Geometry check sheet. Reference: drawing and pictorial views, mm from the part's lowest x, y, z. Give positions to 0.01 mm unless a question says otherwise; leave off trailing zeros. Loops run counter-clockwise (first coordinate to the right, second up) from the corner with the lowest first, then second, coordinate; pieces in that order, holes last. Notation, with made-up numbers: (34, -13) - (71, -13) arc R25 ccw to (71, 17) - close; hole circle Ø8 at (16, -28). An arc over 180 degrees is marked (long way). One line per question, with ' | ' between items. Start each with the question number.
1. Depth check by flat-ended pin: pin 1 Ø2.5 at (x, z) = (50.9, 32) entering from -Y. Enter the tip coordinate at first touch or a pass-through.
2. Section check D-D, the plane y = 0.65. Enter the section's corners in (x, z).
3. Section check B-B, the plane z = 3. Enter the section's corners in (x, y), then the cut area to 3 significant figures.
4. Section check A-A, the plane x = 50.9. Enter the section's corners in (y, z), then the cut area to 3 significant figures.
5. Thickness scan on line 1 along X through (y, z) = (0.7, 32); line 2 along Z through (x, y) = (3.1, 0.6); line 3 along Z through (x, y) = (46.5, 0.4). Record the ranges inside material, lowest first. Write a range as from..to.
6. Section check C-C, the plane x = 3.1. Enter the section's corners in (y, z).
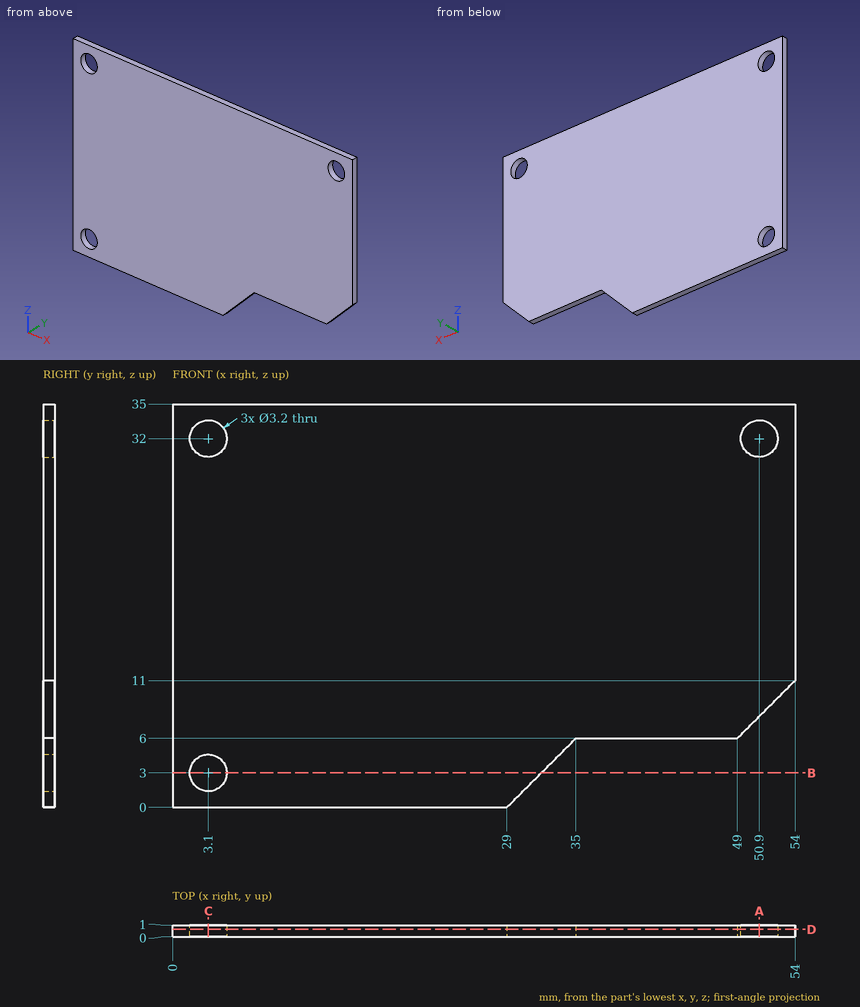
Results list:
1) pin 1: through
2) outline: (0, 0) - (29, 0) - (35, 6) - (49, 6) - (54, 11) - (54, 35) - (0, 35) - close; hole circle Ø3.2 at (3.1, 3); hole circle Ø3.2 at (3.1, 32); hole circle Ø3.2 at (50.9, 32)
3) outline: (0, 0) - (1.5, 0) - (1.5, 1) - (0, 1) - close; (4.7, 0) - (32, 0) - (32, 1) - (4.7, 1) - close | area: 28.8 mm²
4) outline: (0, 7.9) - (1, 7.9) - (1, 30.4) - (0, 30.4) - close; (0, 33.6) - (1, 33.6) - (1, 35) - (0, 35) - close | area: 23.9 mm²
5) line 1: 0..1.5, 4.7..49.3, 52.5..54 | line 2: 0..1.4, 4.6..30.4, 33.6..35 | line 3: 6..35
6) outline: (0, 0) - (1, 0) - (1, 1.4) - (0, 1.4) - close; (0, 4.6) - (1, 4.6) - (1, 30.4) - (0, 30.4) - close; (0, 33.6) - (1, 33.6) - (1, 35) - (0, 35) - close
